from build123d import *

# Parameters (mm, degrees)
F1_DEPTH = 25


with BuildPart() as f1:
    # F0 (on Right) → F1 (new body)
    with BuildSketch(Plane.YZ):
        with BuildLine():
            ThreePointArc((32.1662380939, -32.9784685673), (42.45041522, -17.8943708973), (46.0678441232, 0))
            ThreePointArc((46.0678441232, 0), (43.6151120373, 14.8313271197), (36.5180912177, 28.0833629747))
            Line((36.5180912177, 28.0833629747), (0, 46.0678441232))
            Line((0, 46.0678441232), (-31.7657145821, 33.364436744))
            ThreePointArc((-31.7657145821, 33.364436744), (-45.8389447899, 4.5866548494), (-37.7466590893, -26.4090134188))
            Line((-37.7466590893, -26.4090134188), (-7.6490031363, -45.4283943495))
            ThreePointArc((-7.6490031363, -45.4283943495), (1.0679410721, -46.0554639975), (9.7464507406, -45.0250259313))
            Line((9.7464507406, -45.0250259313), (32.1662380939, -32.9784685673))
        make_face()
        with BuildLine():
            ThreePointArc((36.5180912177, 28.0833629747), (43.6151120373, 14.8313271197), (46.0678441232, 0))
            ThreePointArc((46.0678441232, 0), (42.45041522, -17.8943708973), (32.1662380939, -32.9784685673))
            Line((32.1662380939, -32.9784685673), (93.5423001647, 0))
            Line((93.5423001647, 0), (36.5180912177, 28.0833629747))
        make_face()
        with BuildLine():
            Line((0, 46.0678441232), (36.5180912177, 28.0833629747))
            ThreePointArc((36.5180912177, 28.0833629747), (20.3532095034, 41.3278734641), (0, 46.0678441232))
        make_face()
        with BuildLine():
            ThreePointArc((9.7464507406, -45.0250259313), (21.8047760231, -40.5807590459), (32.1662380939, -32.9784685673))
            Line((32.1662380939, -32.9784685673), (9.7464507406, -45.0250259313))
        make_face()
        with BuildLine():
            Line((-31.7657145821, 33.364436744), (0, 46.0678441232))
            ThreePointArc((0, 46.0678441232), (-17.1058263608, 42.7742558868), (-31.7657145821, 33.364436744))
        make_face()
        with BuildLine():
            ThreePointArc((-31.7657145821, 33.364436744), (-17.1058263608, 42.7742558868), (0, 46.0678441232))
            Line((0, 46.0678441232), (-78.8181275129, 101.4166995883))
            Line((-78.8181275129, 101.4166995883), (-152.4393260479, 46.0678441232))
            Line((-152.4393260479, 46.0678441232), (-93.3580668383, 8.7330770393))
            Line((-93.3580668383, 8.7330770393), (-31.7657145821, 33.364436744))
        make_face()
        with BuildLine():
            Line((0, -50.2619702472), (9.7464507406, -45.0250259313))
            ThreePointArc((9.7464507406, -45.0250259313), (1.0679410721, -46.0554639975), (-7.6490031363, -45.4283943495))
            Line((-7.6490031363, -45.4283943495), (0, -50.2619702472))
        make_face()
        with BuildLine():
            ThreePointArc((-37.7466590893, -26.4090134188), (-45.8389447899, 4.5866548494), (-31.7657145821, 33.364436744))
            Line((-31.7657145821, 33.364436744), (-93.3580668383, 8.7330770393))
            Line((-93.3580668383, 8.7330770393), (-37.7466590893, -26.4090134188))
        make_face()
        with BuildLine():
            Line((0, -50.2619702472), (-7.6490031363, -45.4283943495))
            ThreePointArc((-7.6490031363, -45.4283943495), (-13.1340921063, -44.1558816773), (-18.4229631222, -42.2236982269))
            Line((-18.4229631222, -42.2236982269), (0, -50.2619702472))
        make_face()
        with BuildLine():
            ThreePointArc((-18.4229631222, -42.2236982269), (-13.1340921063, -44.1558816773), (-7.6490031363, -45.4283943495))
            Line((-7.6490031363, -45.4283943495), (-37.7466590893, -26.4090134188))
            ThreePointArc((-37.7466590893, -26.4090134188), (-29.1767489405, -35.6505762004), (-18.4229631222, -42.2236982269))
        make_face()
        with BuildLine():
            ThreePointArc((-18.4229631222, -42.2236982269), (-29.1767489405, -35.6505762004), (-37.7466590893, -26.4090134188))
            Line((-37.7466590893, -26.4090134188), (-93.3580668383, 8.7330770393))
            Line((-93.3580668383, 8.7330770393), (-115.1957064867, 0))
            Line((-115.1957064867, 0), (-18.4229631222, -42.2236982269))
        make_face()
    extrude(amount=F1_DEPTH)


solid = f1.part
Part model, mm, in its own coordinate system. A direction names the side the tool comes from. Give positions to 0.01 mm unless a question says otherwise; leave off trailing zeros. Order: outer loops, then holes, each group sorted by start corner. A loop starts at its lowest first (then second) coordinate and runs counter-clockwise, first axis right, second up. Notation, with made-up numbers: (71, 70.25) - (76, 70.25) arc R22 ccw to (76, 86.25) - close; hole circle Ø3 at (81, 24.25). An arc over 180 degrees is marked (long way). Use a Markdown table: item, result.
1) 3-axis set-ups, long thin cutter, end or side, ignore diameter. For faces 1 (the cylindrical face through (12.325, 21.646, -40.666)), 2 (the flat face through (12.32, -104.12, 4.43)): which of +Z, -Z, +X, -X, +Y, -Y reach the whole face in a straight line?
Checked values:
| item | result |
|---|---|
| face 1 | -Z, +X, -X, +Y |
| face 2 | +X, -X, -Y |
2) Saw through at C-C on z = 2.5. List the corners of the cut face in (x, y).
Checked values:
| item | result |
|---|---|
| outline | (0, -108.94) - (25, -108.94) - (25, 88.47) - (0, 88.47) - close |
3) Flat gauge pins, fed straight in: P1, Ø10, axis at x = 3.5, z = -29, coming from the +Y side; P2, Ø8, axis at x = 14.5, z = 59.5, coming from the +Y side; P3, Ø5, axis at x = 19, y = -74, coming from the -Z side. Where does each tip first touch, or does it go through?
Checked values:
| item | result |
|---|---|
| P1 | y = 48.88 |
| P2 | y = -13.43 |
| P3 | z = -19.07 |
4) Saw through at A-A on x = 13.5. List the corners of the cut face in (y, z).
Checked values:
| item | result |
|---|---|
| outline | (-152.44, 46.07) - (-93.36, 8.73) - (-115.2, 0) - (0, -50.26) - (9.75, -45.03) arc R46.07 ccw to (32.17, -32.98) - (93.54, 0) - (36.52, 28.08) arc R46.07 ccw to (0, 46.07) - (-78.82, 101.42) - close |
5) Saw through at D-D on y = -14. List the corners of the cut face in (x, z).
Checked values:
| item | result |
|---|---|
| outline | (0, -44.15) - (25, -44.15) - (25, 55.9) - (0, 55.9) - close |
6) Probe L1, parallel to Y at x = 4.5, z = 80; L2, parallel to Y at x = 8.5, z = -26; L3, parallel to Z at x = 21, y = 38. List the from-to ranges inside material, lowest first. Write a range as from..to.
Checked values:
| item | result |
|---|---|
| L1 | -107.31..-48.32 |
| L2 | -55.61..45.15 |
| L3 | -29.84..27.35 |
7) Saw through at B-B on y = -112.5. List the corners of the cut face in (x, z).
Checked values:
| item | result |
|---|---|
| outline | (0, -1.18) - (25, -1.18) - (25, 1.08) - (0, 1.08) - close; (0, 20.83) - (25, 20.83) - (25, 76.09) - (0, 76.09) - close |
